Geometry: see drawing. Coordinates: mm, zero at the bounding-box minimum. Give positions to 0.01 mm unless a question says otherwise; leave off trailing zeros. Order: outer loops, then holes, each group sorted by start corner. A loop starts at its lowest first (then second) coordinate and runs counter-clockwise, first axis right, second up. Notation, with made-up numbers: (50, 17) - (104, 17) arc R21 ccw to (104, 33) - close; hole circle Ø9 at (-1, 40). An arc over 180 degrees is marked (long way). One line per question, with ' | ' between items. Start each with the question number.
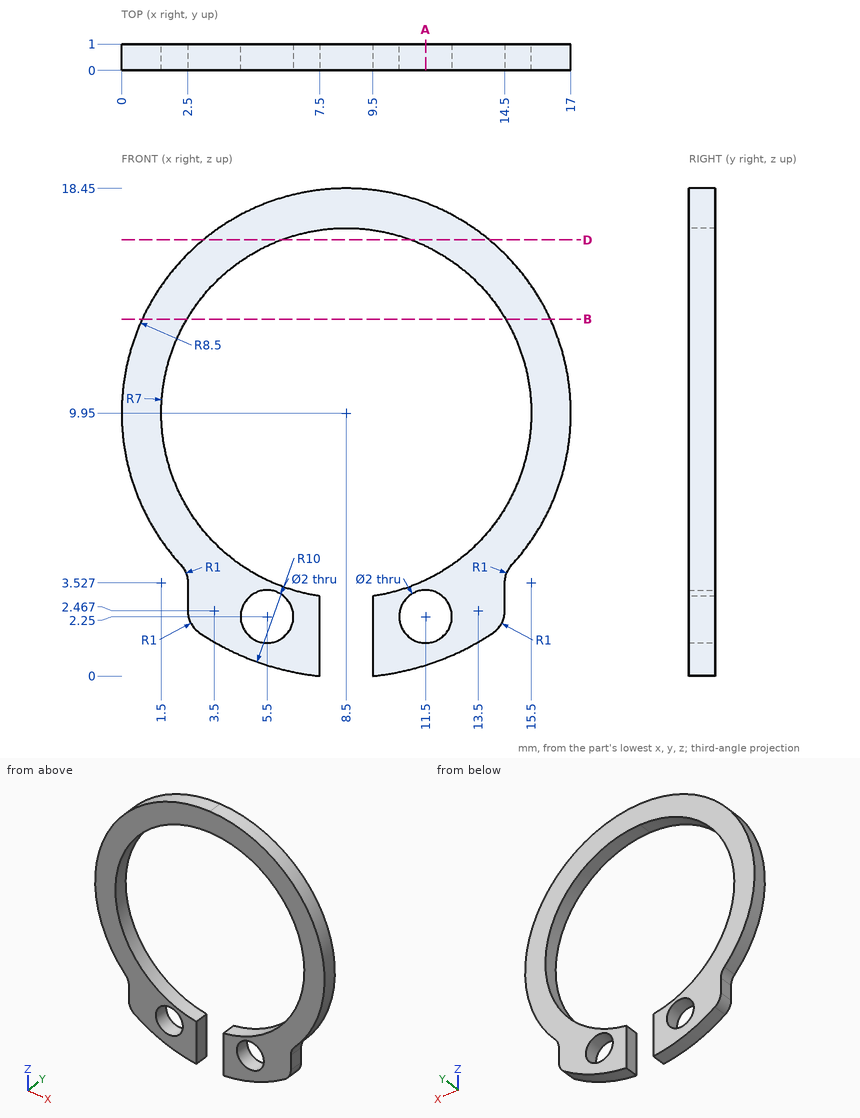
(1) Cut plane D-D, the plane z = 16.5. Return the cut outline in (x, y).
(2) Cut plane A-A, the plane x = 11.5. Give the number of separate pieces and of enclosed holes in the cut face.
(3) Material intervals for line 1 along Z through (x, y) = (10.75, 0.8) (1 decimal); line 2 along X through (y, z) = (0.2, 2.5); line 3 along X through (y, z) = (0.25, 8.75) (1 decimal), sorted ascending. Write a range as from..to.
(4) Cut plane B-B, the plane z = 13.5. Return the cut outline in (x, y).
Results are:
1) outline: (3.08, 0) - (6.03, 0) - (6.03, 1) - (3.08, 1) - close; (10.97, 0) - (13.92, 0) - (13.92, 1) - (10.97, 1) - close
2) separate pieces: 3 | enclosed holes: 0
3) line 1: 0.2..1.6, 2.9..3.3, 16.6..18.1 | line 2: 2.5..4.53, 6.47..7.5, 9.5..10.53, 12.47..14.5 | line 3: 0.1..1.6, 15.4..16.9
4) outline: (0.78, 0) - (2.47, 0) - (2.47, 1) - (0.78, 1) - close; (14.53, 0) - (16.22, 0) - (16.22, 1) - (14.53, 1) - close
